Work out the finished part from the listing and answer in its coordinate system (mm). A direction names the side the tool comes from. Round coordinates to 2 decimals unless told otherwise and drop trailing zeros. Loops run counter-clockwise (first coordinate to the right, second up) from the corner with the lowest first, then second, coordinate; pieces in that order, holes last. Notation, with made-up numbers: (79, -37) - (102, -37) arc R23 cw to (102, -27) - close; hole circle Ø10 at (-20.75, 22.5). An arc over 180 degrees is marked (long way). Answer as CSV lines item,"result". Start each with the question number.
Q1. Straight lines are drawn through the part: L1, parallel to X at y = 2.75, z = -2.25; L2, parallel to X at y = 1.5, z = -2.75; L3, parallel to X at y = 12, z = 2.5. For each, find the intervals that lie inside material, in ascending order. Write a range as [from, to].
Q2. Each of these flat-tipped pins is pushed along its axis until it touches: pin 1 Ø3 at (y, z) = (11, -3.5) entering from -X; pin 2 Ø1 at (x, y) = (14, 12) entering from -Z; pin 3 Ø4.5 at (y, z) = (10.5, 6.5) entering from +X. Where does it stop, or does it pass through?
Q3. Section B-B on y = 11.5 is taken. Write down the section's boundary in (x, z) (3 decimals), then the cut area to 3 significant figures.
Q4. The mould has two halves that part along X. Classify faces 1 (the face through (27.394, 8, 6)), 2 (the face through (4.348, 2.337, 5.83)), 3 (the face through (-37.486, 8, 5)), 4 (the face through (-5, 0, 4)): +X half, -X half, draft (parallel to the pull), parting line (faces both ways), or undercut.
Q5. Section D-D on x = -9.5 is taken. Write down the section's boundary in (y, z), then the cut area to 4 significant figures.
Q6. Section A-A on z = -3.75 is taken. Write down the section's boundary in (x, y), then the cut area to 3 significant figures.
Q7. Section C-C on x = -31 is taken. Write down the section's boundary in (y, z).
Q8. For faces 5 (the face through (-5, 8, 0)), 6 (the face through (-14.223, 10.113, 5.83)), determine the directions among +Z, -Z, +X, -X, +Y, -Y from which every point of the face is accessible in a straight line to the end or side of a thin tool.
```python
from build123d import *

# Parameters (mm, degrees)
BOSS_EXTRUDE1_DEPTH = 17
SKETCH2_R           = 3.175
CUT_EXTRUDE1_DEPTH  = 18
SKETCH4_R           = 1
CUT_EXTRUDE3_DEPTH  = 18.75
FILLET1_R           = 1


with BuildPart() as part:
    # Sketch1 → Boss-Extrude1 (new body)
    with BuildSketch(Plane(origin=(0, 0, 0), x_dir=(1, 0, 0), z_dir=(0, 1, 0))):
        with BuildLine():
            Line((-24.985807588, 0), (15.020468055, 0))
            ThreePointArc((15.020468055, 0), (21.898649068, 6.218350956), (27.394192412, -1.25))
            Line((27.394192412, -1.25), (27.394192412, -11.5))
            Line((27.394192412, -11.5), (-37.485807588, -11.5))
            Line((-37.485807588, -11.5), (-37.485807588, 0))
            ThreePointArc((-37.485807588, 0), (-31.235807588, 6.25), (-24.985807588, 0))
        make_face()
    extrude(amount=BOSS_EXTRUDE1_DEPTH)

    # Sketch2 → Cut-Extrude1 (cut, through all)
    with BuildSketch(Plane(origin=(0, 17, 0), x_dir=(1, 0, 0), z_dir=(0, 1, 0))):
        with Locations((-31.235807588, 0)):
            Circle(SKETCH2_R)
        with Locations((21.270468055, 0)):
            Circle(SKETCH2_R)
    extrude(amount=-CUT_EXTRUDE1_DEPTH, mode=Mode.SUBTRACT)

    # Sketch4 → Cut-Extrude3 (cut, through all)
    with BuildSketch(Plane.XY.offset(11.5)):
        with Locations((-13.485807588, 9.437)):
            Circle(SKETCH4_R)
        with Locations((3.394192412, 2.037)):
            Circle(SKETCH4_R)
    extrude(amount=-CUT_EXTRUDE3_DEPTH, mode=Mode.SUBTRACT)

    # Fillet1
    fillet1_edges = [part.edges().sort_by_distance(p)[0] for p in [
        (27.394192412, 8.5, 11.5),
        (-37.485807588, 8.5, 11.5),
    ]]
    fillet(fillet1_edges, radius=FILLET1_R)


solid = part.part
```
Findings:
1,L1,"x = [-37.07, -33.48], [-29, -25.4], [15.44, 19.03], [23.51, 27.1]"
1,L2,"x = [-36.85, -32.82], [-29.65, -25.62], [15.66, 19.68], [22.86, 26.88]"
1,L3,"x = [-37.49, -33.19], [-29.28, 19.31], [23.23, 27.39]"
2,pin 1,"stops at x = -37.16"
2,pin 2,"stops at z = 0"
2,pin 3,"stops at x = 27.39"
3,outline,"(-37.486, 0) arc R6.25 ccw to (-24.986, 0) - (15.02, 0) arc R6.25 ccw (long way) to (27.394, 1.25) - (27.394, 10.5) arc R1 ccw to (26.394, 11.5) - (-36.486, 11.5) arc R1 ccw to (-37.486, 10.5) - close; hole circle Ø6.35 at (-31.236, 0); hole circle Ø6.35 at (21.27, 0)"
3,area,"805 mm^2"
4,face 1,"+X half"
4,face 2,"undercut"
4,face 3,"-X half"
4,face 4,"draft"
5,outline,"(0, 0) - (17, 0) - (17, 11.5) - (0, 11.5) - close"
5,area,"195.5 mm^2"
6,outline,"(-36.24, 0) - (-26.24, 0) - (-26.24, 17) - (-36.24, 17) - close; (16.27, 0) - (26.27, 0) - (26.27, 17) - (16.27, 17) - close"
6,area,"340 mm^2"
7,outline,"(0, -6.25) - (17, -6.25) - (17, -3.17) - (0, -3.17) - close; (0, 3.17) - (17, 3.17) - (17, 11.5) - (0, 11.5) - close"
8,face 5,"-Z, +Y, -Y"
8,face 6,"+Z, -Z"
